Answer from the drawing. Dimensions are ordinates in mm from the lowest x, y and z of the part. A direction names the side the tool comes from. Round coordinates to 2 decimals unless told otherwise and drop trailing zeros. Write each loop counter-clockwise with the first axis right and the second up, starting at its lowest first coordinate (ties: lowest second). Pieces come first, ordered by that corner, then holes.
1. Straight lines are drawn through the part: probe 1 along X at (y, z) = (5.75, 1.2); probe 2 along Y at (x, z) = (2, 0.65); probe 3 along X at (y, z) = (6.5, 0.4) (1 decimal). For each, find the intervals that lie inside material, in ascending order.
2. Find section A-A (x = 2). Write down the section's boundary in (y, z).
3. Find section D-D (y = 0.75). Write down the section's boundary in (x, z) (1 decimal), and give its area (3 significant figures).
4. A tool of negligible diameter and unlimited length cuts with its end or side. For the marked faces 3 and 4, from which of +Z, -Z, +X, -X, +Y, -Y can it reach the whole face along a straight path? Write none if from no direction.
5. Find section C-C (z = 0.4). Write down the section's boundary in (x, y), and give its area (3 significant figures).
6. A flat-ended cylindrical pin translates along its axis: pin 1 Ø0.8 at (x, z) = (16.5, 1) entering from +Y. Find the tip coordinate at first contact, or state that the pin passes through.
7. Determine the mould class of the marked faces 1 and 2 for opening direction X: pulls with the +X half, pulls with the -X half, needs draft (parallel to the pull), parting line crosses it, or undercut.
8. Find section B-B (y = 5.25). Write down the section's boundary in (x, z).
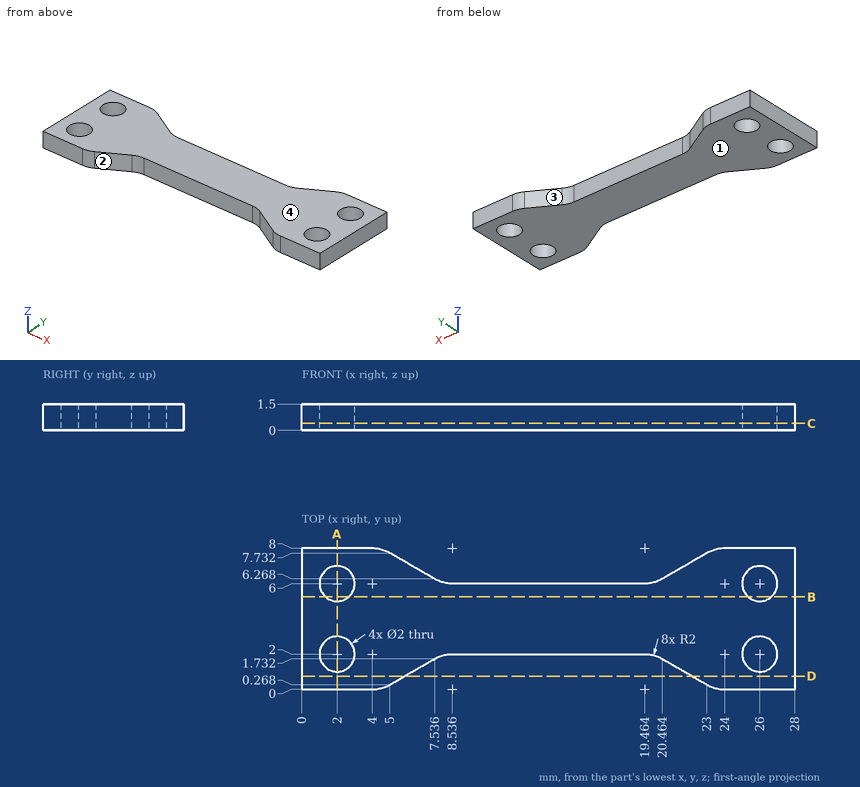
Worked answers:
1. probe 1: x = 0 to 1.03, 2.97 to 25.03, 26.97 to 28
1. probe 2: y = 0 to 1, 3 to 5, 7 to 8
1. probe 3: x = 0 to 1.1, 2.9 to 7.1, 20.9 to 25.1, 26.9 to 28
2. outline: (0, 0) - (1, 0) - (1, 1.5) - (0, 1.5) - close; (3, 0) - (5, 0) - (5, 1.5) - (3, 1.5) - close; (7, 0) - (8, 0) - (8, 1.5) - (7, 1.5) - close
3. outline: (0, 0) - (5.8, 0) - (5.8, 1.5) - (0, 1.5) - close; (22.2, 0) - (28, 0) - (28, 1.5) - (22.2, 1.5) - close
3. area: 17.5 mm2
4. face 3: +Z, -Z, +Y
4. face 4: +Z, +X, -X, +Y, -Y
5. outline: (0, 0) - (4, 0) arc R2 ccw to (5, 0.27) - (7.54, 1.73) arc R2 cw to (8.54, 2) - (19.46, 2) arc R2 cw to (20.46, 1.73) - (23, 0.27) arc R2 ccw to (24, 0) - (28, 0) - (28, 8) - (24, 8) arc R2 ccw to (23, 7.73) - (20.46, 6.27) arc R2 cw to (19.46, 6) - (8.54, 6) arc R2 cw to (7.54, 6.27) - (5, 7.73) arc R2 ccw to (4, 8) - (0, 8) - close; hole circle Ø2 at (2, 2); hole circle Ø2 at (2, 6); hole circle Ø2 at (26, 2); hole circle Ø2 at (26, 6)
5. area: 150 mm2
6. pin 1: stops at y = 6
7. face 1: needs draft
7. face 2: undercut
8. outline: (0, 0) - (1.34, 0) - (1.34, 1.5) - (0, 1.5) - close; (2.66, 0) - (25.34, 0) - (25.34, 1.5) - (2.66, 1.5) - close; (26.66, 0) - (28, 0) - (28, 1.5) - (26.66, 1.5) - close
